Geometry check sheet. Reference: the model listing, model coordinates, mm. Give positions to 0.01 mm unless a question says otherwise; leave off trailing zeros. Loops run counter-clockwise (first coordinate to the right, second up) from the corner with the lowest first, then second, coordinate; pieces in that order, holes last. Notation, with made-up numbers: (-6, -32) -> (-2, -32) arc R36 ccw to (-2, 5) -> close; hole circle Ø3 at (-16, 25.25). An arc over 180 degrees is marked (long way). Write item = value, one per line. Start each with the question number.
```python
from build123d import *

# Parameters (mm, degrees)
CROQUIS1_R              = 100
SALIENTE_EXTRUIR1_DEPTH = 3
CROQUIS3_R              = 120
CORTAR_EXTRUIR1_DEPTH   = 3
CORTAR_EXTRUIR6_DEPTH   = 10
CROQUIS12_R             = 1.5
CORTAR_EXTRUIR7_DEPTH   = 142.453172464
CROQUIS9_R              = 1.5
CROQUIS9_W              = 4.5
CROQUIS9_H              = 8
CROQUIS9_W_2            = 8
CROQUIS9_H_2            = 4.5
CORTAR_EXTRUIR5_DEPTH   = 10


with BuildPart() as part:
    # Croquis1 → Saliente-Extruir1 (new body)
    with BuildSketch(Plane.XY):
        Circle(CROQUIS1_R)
    extrude(amount=SALIENTE_EXTRUIR1_DEPTH)

    # Croquis3 → Cortar-Extruir1 (cut)
    with BuildSketch(Plane.XY.offset(3)):
        with Locations((190, 0)):
            Circle(CROQUIS3_R)
    extrude(amount=-CORTAR_EXTRUIR1_DEPTH, mode=Mode.SUBTRACT)

    # Croquis5 → Cortar-Extruir6 (cut)
    with BuildSketch(Plane.XY.offset(3)):
        Polygon((-58.336309448, -83.085046789), (-83.085046789, -58.336309448), (-65.40737726, -40.658639918), (-40.658639918, -65.40737726), align=None)
        Polygon((-83.085046789, 58.336309448), (-58.336309448, 83.085046789), (-40.658639918, 65.40737726), (-65.40737726, 40.658639918), align=None)
        Polygon((58.336309448, -83.085046789), (83.085046789, -58.336309448), (65.40737726, -40.658639918), (40.658639918, -65.40737726), align=None)
        Polygon((58.336309448, 83.085046789), (83.085046789, 58.336309448), (65.40737726, 40.658639918), (40.658639918, 65.40737726), align=None)
    extrude(amount=-CORTAR_EXTRUIR6_DEPTH, mode=Mode.SUBTRACT)

    # Croquis12 → Cortar-Extruir7 (cut, through all)
    with BuildSketch(Plane.XY.offset(3)):
        with Locations((-63.604254904, -36.804908024)):
            Circle(CROQUIS12_R)
        with Locations((-36.804907897, -63.604255031)):
            Circle(CROQUIS12_R)
        with Locations((-47.666068056, -20.866721176)):
            Circle(CROQUIS12_R)
        with Locations((-20.866721049, -47.666068183)):
            Circle(CROQUIS12_R)
        with Locations(Location((47.666068183, 20.866721049, 0), (0, 0, 180))):
            Circle(CROQUIS12_R)
        with Locations(Location((20.866721176, 47.666068056, 0), (0, 0, 180))):
            Circle(CROQUIS12_R)
        with Locations(Location((63.604255031, 36.804907897, 0), (0, 0, 180))):
            Circle(CROQUIS12_R)
        with Locations(Location((36.804908024, 63.604254904, 0), (0, 0, 180))):
            Circle(CROQUIS12_R)
        with Locations((20.866721325, -47.666067908)):
            Circle(CROQUIS12_R)
        with Locations((47.666068332, -20.866720901)):
            Circle(CROQUIS12_R)
        with Locations((63.60425518, -36.804907749)):
            Circle(CROQUIS12_R)
        with Locations((36.804908173, -63.604254756)):
            Circle(CROQUIS12_R)
        with Locations(Location((-63.604254756, 36.804908173, 0), (0, 0, 180))):
            Circle(CROQUIS12_R)
        with Locations(Location((-36.804907749, 63.60425518, 0), (0, 0, 180))):
            Circle(CROQUIS12_R)
        with Locations(Location((-20.866720901, 47.666068332, 0), (0, 0, 180))):
            Circle(CROQUIS12_R)
        with Locations(Location((-47.666067908, 20.866721325, 0), (0, 0, 180))):
            Circle(CROQUIS12_R)
    extrude(amount=-CORTAR_EXTRUIR7_DEPTH, mode=Mode.SUBTRACT)

    # Croquis9 → Cortar-Extruir5 (cut)
    with BuildSketch(Plane.XY.offset(3)):
        with Locations((66.9, -4)):
            Circle(CROQUIS9_R)
        with Locations((30.9, 4)):
            Circle(CROQUIS9_R)
        with Locations((66.9, 4)):
            Circle(CROQUIS9_R)
        with Locations((30.9, -4)):
            Circle(CROQUIS9_R)
        with Locations((-91.190074744, 4)):
            Circle(CROQUIS9_R)
        with Locations((-91.190074744, -4)):
            Circle(CROQUIS9_R)
        with Locations((-55.190074744, 4)):
            Circle(CROQUIS9_R)
        with Locations((-55.190074744, -4)):
            Circle(CROQUIS9_R)
        with Locations((-4, 85)):
            Circle(CROQUIS9_R)
        with Locations((4, 85)):
            Circle(CROQUIS9_R)
        with Locations((-4, 49)):
            Circle(CROQUIS9_R)
        with Locations((4, 49)):
            Circle(CROQUIS9_R)
        with Locations((-4, -49)):
            Circle(CROQUIS9_R)
        with Locations((4, -49)):
            Circle(CROQUIS9_R)
        with Locations((4, -85)):
            Circle(CROQUIS9_R)
        with Locations((-4, -85)):
            Circle(CROQUIS9_R)
        with Locations((36.15, 0)):
            Rectangle(CROQUIS9_W, CROQUIS9_H)
        with Locations((0, -54.25)):
            Rectangle(CROQUIS9_W_2, CROQUIS9_H_2)
        with Locations((-60.440074744, 0)):
            Rectangle(CROQUIS9_W, CROQUIS9_H)
        with Locations((0, 54.25)):
            Rectangle(CROQUIS9_W_2, CROQUIS9_H_2)
    extrude(amount=-CORTAR_EXTRUIR5_DEPTH, mode=Mode.SUBTRACT)


solid = part.part
```
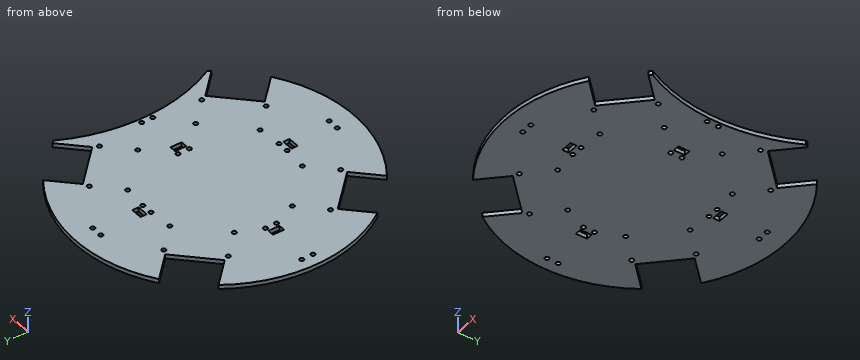
1) Thickness scan on line 1 (Y direction, x = 36.5, z = 2.6); line 2 (Y direction, x = -46, z = 1.5); line 3 (X direction, y = -62.5, z = 1.8). Record the ranges inside material, lowest first.
2) Section check A-A (y = 16). Enter the section's corners in (x, z).
3) Depth check by flat-ended pin: pin 1 Ø4 at (x, y) = (22.5, -42) entering from -Z. Enter the tip coordinate at first touch or a pass-through.
4) Section check B-B (z = 1.75). Give the number of separate pieces and of enclosed holes in the cut face, plus the area to 3 significant figures.
Check result:
q1.line_1 = -93.1 to -65.07, -62.14 to -4, 4 to 62.14, 65.07 to 93.1
q1.line_2 = -88.79 to -70.75, -60.07 to 60.07, 70.75 to 88.79
q1.line_3 = -43.57 to -37.82, -35.79 to 35.79, 37.82 to 43.57
q2.outline = (-98.71, 0) -> (71.07, 0) -> (71.07, 3) -> (-98.71, 3) -> close
q3.pin_1 = 0
q4.separate_pieces = 1
q4.enclosed_holes = 36
q4.area = 25,400 mm2
